```python
from build123d import *

# Parameters (mm, degrees)
CROQUIS1_W              = 50.8
CROQUIS1_H              = 50.8
CROQUIS1_W_2            = 44.8
CROQUIS1_H_2            = 44.8
SALIENTE_EXTRUIR1_DEPTH = 300
CROQUIS2_R              = 6.35
CORTAR_EXTRUIR1_DEPTH   = 306.32900288
CROQUIS3_R              = 6.35
CORTAR_EXTRUIR2_DEPTH   = 70


with BuildPart() as part:
    # Croquis1 → Saliente-Extruir1 (new, symmetric)
    with BuildSketch(Plane.XY):
        Rectangle(CROQUIS1_W, CROQUIS1_H)
        Rectangle(CROQUIS1_W_2, CROQUIS1_H_2, mode=Mode.SUBTRACT)
    extrude(amount=SALIENTE_EXTRUIR1_DEPTH, both=True)

    # Croquis2 → Cortar-Extruir1 (cut, through all)
    with BuildSketch(Plane(origin=(25.4, 0, 0), x_dir=(0, 0, -1), z_dir=(1, 0, 0))):
        with Locations(Location((285, 0, 0), (0, 0, 270))):
            Circle(CROQUIS2_R)
    extrude(amount=-CORTAR_EXTRUIR1_DEPTH, mode=Mode.SUBTRACT)

    # Croquis3 → Cortar-Extruir2 (cut)
    with BuildSketch(Plane(origin=(0, 25.4, 0), x_dir=(1, 0, 0), z_dir=(0, 1, 0))):
        with Locations(Location((0, -273, 0), (0, 0, 270))):
            Circle(CROQUIS3_R)
    extrude(amount=-CORTAR_EXTRUIR2_DEPTH, mode=Mode.SUBTRACT)


solid = part.part
```
Check sheet for the modelled part. Datum: model origin and axes. Units: mm. A direction names the side the tool comes from. Round coordinates to 2 decimals unless told otherwise and drop trailing zeros. Write each loop counter-clockwise with the first axis right and the second up, starting at its lowest first coordinate (ties: lowest second). Pieces come first, ordered by that corner, then holes. Notation, with made-up numbers: (30, 32) -> (52, 32) arc R21 cw to (52, 53) -> close; hole circle Ø6 at (4.25, 40). An arc over 180 degrees is marked (long way). Put each result on its own line as item: value.
(1) Sectioned sample at B-B (x = 0). Enter the section's corners in (y, z), plus the area to 3 significant figures.
Values found:
outline: (-25.4, -300) -> (-22.4, -300) -> (-22.4, 266.65) -> (-25.4, 266.65) -> close; (-25.4, 279.35) -> (-22.4, 279.35) -> (-22.4, 300) -> (-25.4, 300) -> close; (22.4, -300) -> (25.4, -300) -> (25.4, 266.65) -> (22.4, 266.65) -> close; (22.4, 279.35) -> (25.4, 279.35) -> (25.4, 300) -> (22.4, 300) -> close
area: 3,520 mm^2
(2) Tool access check on faces 5 (the face through (-23.9, 0.8, -291.3)), 6 (the face through (0, -22.4, 4)). Record the directions out of +Z, -Z, +X, -X, +Y, -Y that give a thin tool (end or side, any length) a straight path to the whole face; none if there is none.
Values found:
face 5: +X, -X
face 6: +Z, -Z
(3) Mould release check, pull along Y, two halves, no side actions. Record for faces 1 (the face through (-25.4, 0, 4)), 2 (the face through (0, 22.4, 4)), 3 (the face through (0, 25.4, 4)), 4 (the face through (0, -25.4, 4)): released by +Y, released by -Y, zero draft, split by the parting line, or undercut.
Values found:
face 1: zero draft
face 2: undercut
face 3: released by +Y
face 4: released by -Y
(4) Sectioned sample at C-C (z = -72.5). Enter the section's corners in (x, y), plus the area to 3 significant figures.
Values found:
outline: (-25.4, -25.4) -> (25.4, -25.4) -> (25.4, 25.4) -> (-25.4, 25.4) -> close; hole (-22.4, -22.4) -> (22.4, -22.4) -> (22.4, 22.4) -> (-22.4, 22.4) -> close
area: 574 mm^2
(5) Sectioned sample at A-A (y = 0). Enter the section's corners in (x, z), plus the area to 3 significant figures.
Values found:
outline: (-25.4, -300) -> (-22.4, -300) -> (-22.4, -291.35) -> (-25.4, -291.35) -> close; (-25.4, -278.65) -> (-22.4, -278.65) -> (-22.4, 300) -> (-25.4, 300) -> close; (22.4, -300) -> (25.4, -300) -> (25.4, -291.35) -> (22.4, -291.35) -> close; (22.4, -278.65) -> (25.4, -278.65) -> (25.4, 300) -> (22.4, 300) -> close
area: 3,520 mm^2
(6) Sectioned sample at D-D (z = 273). Enter the section's corners in (x, y), plus the area to 3 significant figures.
Values found:
outline: (-25.4, -25.4) -> (-6.35, -25.4) -> (-6.35, -22.4) -> (-22.4, -22.4) -> (-22.4, 22.4) -> (-6.35, 22.4) -> (-6.35, 25.4) -> (-25.4, 25.4) -> close; (6.35, -25.4) -> (25.4, -25.4) -> (25.4, 25.4) -> (6.35, 25.4) -> (6.35, 22.4) -> (22.4, 22.4) -> (22.4, -22.4) -> (6.35, -22.4) -> close
area: 497 mm^2
(7) Material ranges on line 1 (Y direction, x = 8.5, z = -169); line 2 (Y direction, x = 23.1, z = -285); line 3 (Z direction, x = -24, y = 0), recorded low to high.
Values found:
line 1: y = -25.4 to -22.4, 22.4 to 25.4
line 2: y = -25.4 to -6.35, 6.35 to 25.4
line 3: z = -300 to -291.35, -278.65 to 300
